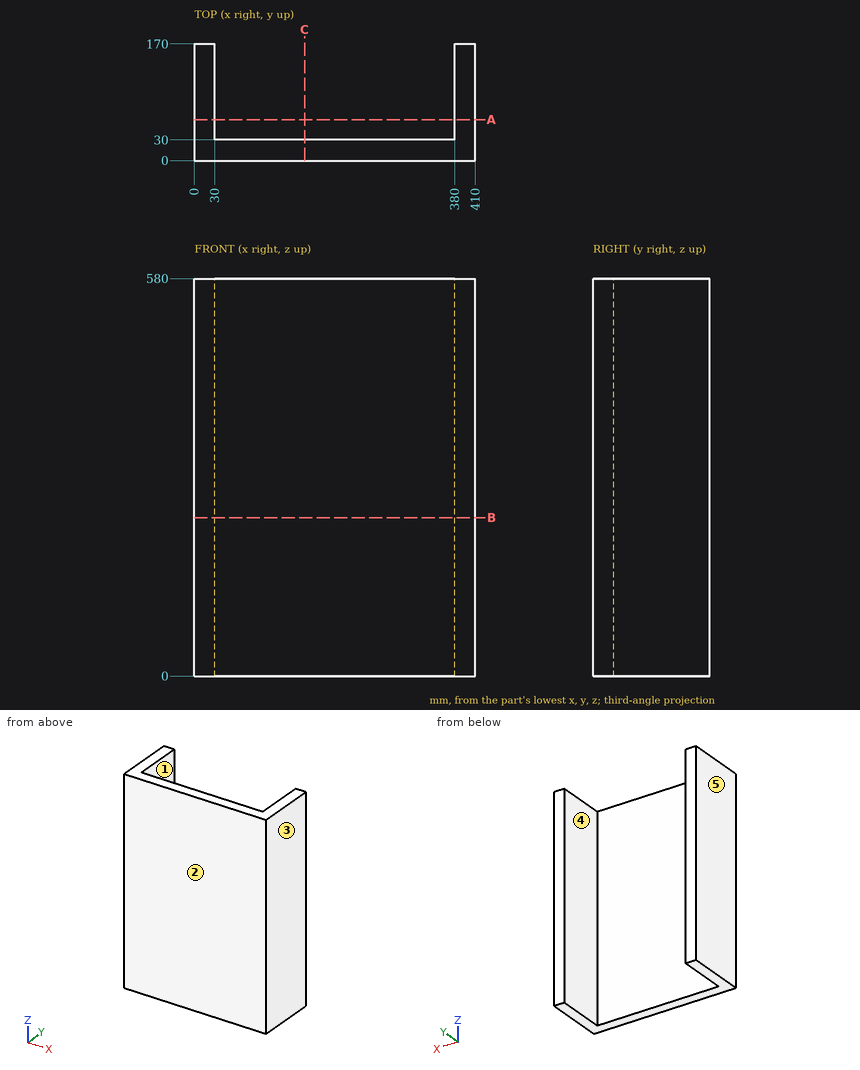
Part print with two shaded views. Sizes in mm from the minimum x, y, z corner. A direction names the side the tool comes from. Round coordinates to 2 decimals unless told otherwise and drop trailing zeros. Write each loop counter-clockwise with the first axis right and the second up, starting at its lowest first coordinate (ties: lowest second). Pieces come first, ordered by that corner, then holes. Notation, with made-up numbers: (-21, 14) -> (23, 14) arc R22 cw to (23, 28) -> close; hole circle Ø9 at (82.5, -7). An arc over 180 degrees is marked (long way). Put each result on its own line as item: value.
Item 1: Wall check: probe 1 along X at (y, z) = (68.5, 312); probe 2 along Y at (x, z) = (45, 229.5). Give the ranges that are in metal, low to high. Write a range as from..to.
Here are the results:
probe 1: x = 0..30, 380..410
probe 2: y = 0..30
Item 2: Two-plate mould, pull along X, no slides. Class the marked faces 3, 4 and 5: pulls with the +X half, pulls with the -X half, needs draft (parallel to the pull), parting line crosses it, or undercut.
Here are the results:
face 3: pulls with the +X half
face 4: undercut
face 5: pulls with the -X half
Item 3: Slice it at C-C, the plane x = 161. Give the cut face in (y, z), plus the area to 3 significant figures.
Here are the results:
outline: (0, 0) -> (30, 0) -> (30, 580) -> (0, 580) -> close
area: 17,400 mm^2
Item 4: Flat gauge pin, fed straight in: P1, Ø6, axis at x = 42.5, z = 380, coming from the +Y side. Where does the tip first touch, or does it go through?
Here are the results:
P1: stops at y = 30
Item 5: Tool access for the marked faces 1 and 2: list every direction of +Z, -Z, +X, -X, +Y, -Y with a clear straight run to the whole face (end or side of a thin tool).
Here are the results:
face 1: +Z, -Z, +Y
face 2: +Z, -Z, +X, -X, -Y
Item 6: Slice it at A-A, the plane y = 59.5. Give the cut face in (x, z).
Here are the results:
outline: (0, 0) -> (30, 0) -> (30, 580) -> (0, 580) -> close; (380, 0) -> (410, 0) -> (410, 580) -> (380, 580) -> close
Item 7: Slice it at B-B, the plane z = 231. Give the cut face in (x, y).
Here are the results:
outline: (0, 0) -> (410, 0) -> (410, 170) -> (380, 170) -> (380, 30) -> (30, 30) -> (30, 170) -> (0, 170) -> close
